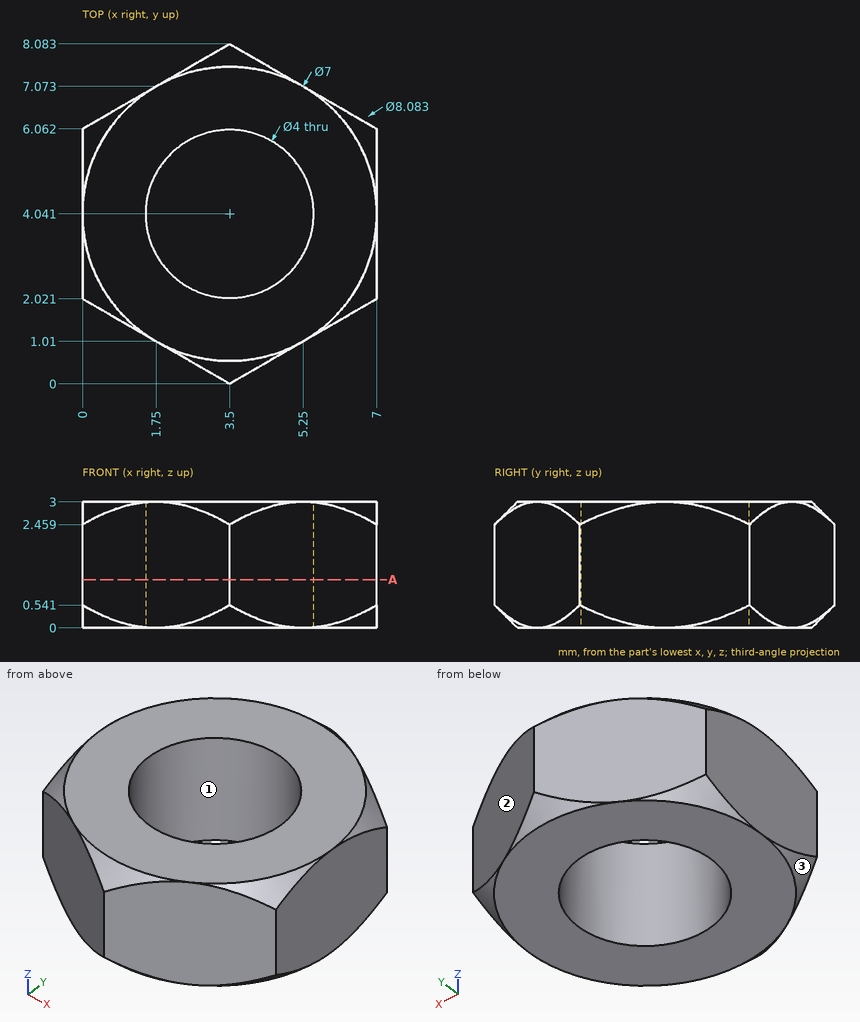
The figure shows three views and two pictorial views of one solid part (mm, origin at its lowest corner). Answer the questions. Coordinates: 2 decimals unless noted, no trailing zeros. Loops run counter-clockwise (first coordinate to the right, second up) from the corner with the lowest first, then second, coordinate; pieces in that order, holes last.
1) Determine the mould class of the marked faces 1, 2 and 3 for opening direction Y: pulls with the +Y half, pulls with the -Y half, needs draft (parallel to the pull), parting line crosses it, or undercut.
2) Find the intervals of material crossed by L1, parallel to X at y = 4, z = 1.1; L2, parallel to X at y = 5.5, z = 0.75; L3, parallel to Y at x = 2.25, z = 0.7 (1 decimal), in increasing order.
3) Find section A-A on z = 1.15. Write down the section's boundary in (x, y).
4) A flat-ended cylindrical pin translates along its axis: pin 1 Ø2 at (x, y) = (2.5, 3) entering from +Z. Find the tip coordinate at first contact, or state that the pin passes through.
Values:
1. face 1: undercut
1. face 2: pulls with the +Y half
1. face 3: pulls with the -Y half
2. L1: x = 0 to 1.5, 5.5 to 7
2. L2: x = 0 to 2.13, 4.87 to 7
2. L3: y = 0.7 to 2.5, 5.6 to 7.4
3. outline: (0, 2.02) - (3.5, 0) - (7, 2.02) - (7, 6.06) - (3.5, 8.08) - (0, 6.06) - close; hole circle Ø4 at (3.5, 4.04)
4. pin 1: stops at z = 3
